Here's how the part is built. I have some questions about the finished solid (model axes, mm). Face numbers are marked on the shaded views. A direction names the side the tool comes from. Give positions to 0.01 mm unless a question says otherwise; leave off trailing zeros. Write each loop counter-clockwise with the first axis right and the second up, starting at its lowest first coordinate (ties: lowest second). Pieces come first, ordered by that corner, then holes. Notation, with made-up numbers: (80.5, -33.5) - (110.5, -33.5) arc R13 ccw to (110.5, -13.5) - close; hole circle Ø1 at (38.5, 16). An arc over 180 degrees is marked (long way). Use a Markdown table: item, result.
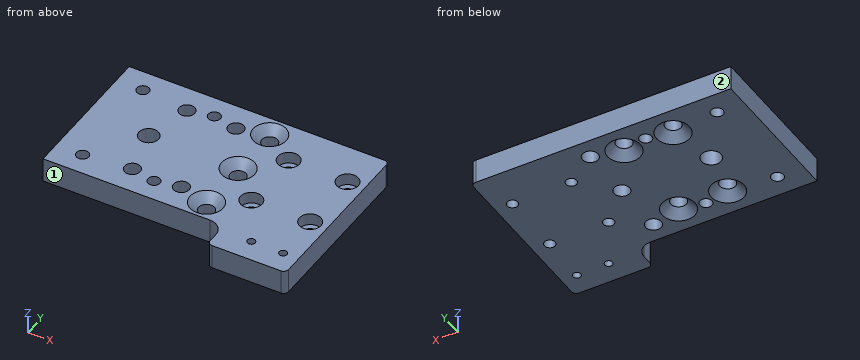
```python
from build123d import *

# Parameters (mm, degrees)
SCHIZZO1_W                                           = 52
SCHIZZO1_H                                           = 30
ESTRUSIONE_ESTRUSIONE1_DEPTH                         = 5
FORO_LAMATO_PER_VITE_M2_A_TESTA_CILINDRI_D           = 2.2
FORO_LAMATO_PER_VITE_M2_A_TESTA_CILINDRI_DEPTH       = 8.5
FORO_LAMATO_PER_VITE_M2_A_TESTA_CILINDRI_CBORE_D     = 4.4
FORO_LAMATO_PER_VITE_M2_A_TESTA_CILINDRI_CBORE_DEPTH = 2.4
FORO_LAMATO_PER_VITE_M2_A_TESTA_CILINDRI_TIP         = 0.660946681
FORO_SVASATO_PER_VITE_M3_1_D                         = 3.2
FORO_SVASATO_PER_VITE_M3_1_DEPTH                     = 8.5
FORO_SVASATO_PER_VITE_M3_1_CSINK_D                   = 6.72
FORO_SVASATO_PER_VITE_M3_1_CSINK_ANGLE               = 90
FORO_SVASATO_PER_VITE_M3_1_TIP                       = 0.96137699
FORO_4_0_4_1_D                                       = 4
FORO_4_0_4_1_DEPTH                                   = 8.5
FORO_4_0_4_1_TIP                                     = 1.201721238
FORO_FILETTATO_M3_1_D                                = 2.5
FORO_FILETTATO_M3_1_DEPTH                            = 8.5
FORO_FILETTATO_M3_1_TIP                              = 0.751075774
FORO_SVASATO_PER_VITE_M3_2_D                         = 3.2
FORO_SVASATO_PER_VITE_M3_2_CSINK_D                   = 6.72
FORO_SVASATO_PER_VITE_M3_2_CSINK_ANGLE               = 90
SCHIZZO11_W                                          = 15
SCHIZZO11_H                                          = 5
ESTRUSIONE_ESTRUSIONE2_DEPTH                         = 6
FORO_FILETTATO_M2_1_D                                = 1.6
FORO_FILETTATO_M2_1_DEPTH                            = 6
FORO_FILETTATO_M2_1_TIP                              = 0.480688495
SCHIZZO14_W                                          = 1
SCHIZZO14_H                                          = 5
ESTRUSIONE_ESTRUSIONE3_DEPTH                         = 36
RACCORDO1_R                                          = 1
RACCORDO2_R                                          = 3


with BuildPart() as part:
    # Schizzo1 → Estrusione-Estrusione1 (new body)
    with BuildSketch(Plane.XY):
        Rectangle(SCHIZZO1_W, SCHIZZO1_H)
    extrude(amount=ESTRUSIONE_ESTRUSIONE1_DEPTH)

    # Foro lamato per Vite M2 a testa cilindrica-1
    with Locations(Plane(origin=(11.5, 6.5, 5), x_dir=(1, 0, 0), z_dir=(0, 0, 1))):
        with Locations((0, 0), (12, 0), (0, -13), (12, -13)):
            CounterBoreHole(FORO_LAMATO_PER_VITE_M2_A_TESTA_CILINDRI_D / 2, FORO_LAMATO_PER_VITE_M2_A_TESTA_CILINDRI_CBORE_D / 2, FORO_LAMATO_PER_VITE_M2_A_TESTA_CILINDRI_CBORE_DEPTH, depth=FORO_LAMATO_PER_VITE_M2_A_TESTA_CILINDRI_DEPTH)
            with Locations((0, 0, -(FORO_LAMATO_PER_VITE_M2_A_TESTA_CILINDRI_DEPTH + FORO_LAMATO_PER_VITE_M2_A_TESTA_CILINDRI_TIP / 2))):  # 118° drill point
                Cone(0, FORO_LAMATO_PER_VITE_M2_A_TESTA_CILINDRI_D / 2, FORO_LAMATO_PER_VITE_M2_A_TESTA_CILINDRI_TIP, mode=Mode.SUBTRACT)

    # Foro svasato per Vite M3-1
    with Locations(Plane(origin=(0, 0, 0), x_dir=(-1, 0, 0), z_dir=(0, 0, -1))):
        with Locations((11, -9.5), (1, -9.5), (11, 9.5), (1, 9.5)):
            CounterSinkHole(FORO_SVASATO_PER_VITE_M3_1_D / 2, FORO_SVASATO_PER_VITE_M3_1_CSINK_D / 2, depth=FORO_SVASATO_PER_VITE_M3_1_DEPTH, counter_sink_angle=FORO_SVASATO_PER_VITE_M3_1_CSINK_ANGLE)
            with Locations((0, 0, -(FORO_SVASATO_PER_VITE_M3_1_DEPTH + FORO_SVASATO_PER_VITE_M3_1_TIP / 2))):  # 118° drill point
                Cone(0, FORO_SVASATO_PER_VITE_M3_1_D / 2, FORO_SVASATO_PER_VITE_M3_1_TIP, mode=Mode.SUBTRACT)

    # Foro Ø4.0 (4)-1
    with Locations(Plane(origin=(-13.23, 0, 5), x_dir=(1, 0, 0), z_dir=(0, 0, 1))):
        with Locations((0, 0)):
            Hole(FORO_4_0_4_1_D / 2, depth=FORO_4_0_4_1_DEPTH)
            with Locations((0, 0, -(FORO_4_0_4_1_DEPTH + FORO_4_0_4_1_TIP / 2))):  # 118° drill point
                Cone(0, FORO_4_0_4_1_D / 2, FORO_4_0_4_1_TIP, mode=Mode.SUBTRACT)

    # Foro filettato M3-1
    with Locations(Plane(origin=(-20.56, 10.5, 5), x_dir=(1, 0, 0), z_dir=(0, 0, 1))):
        with Locations((0, 0), (14.56, 0), (14.56, -21), (0, -21)):
            Hole(FORO_FILETTATO_M3_1_D / 2, depth=FORO_FILETTATO_M3_1_DEPTH)
            with Locations((0, 0, -(FORO_FILETTATO_M3_1_DEPTH + FORO_FILETTATO_M3_1_TIP / 2))):  # 118° drill point
                Cone(0, FORO_FILETTATO_M3_1_D / 2, FORO_FILETTATO_M3_1_TIP, mode=Mode.SUBTRACT)

    # Foro svasato per Vite M3-2 (through all)
    with Locations(Plane(origin=(5, 11, 5), x_dir=(1, 0, 0), z_dir=(0, 0, 1))):
        with Locations((0, 0), (0, -11), (0, -22)):
            CounterSinkHole(FORO_SVASATO_PER_VITE_M3_2_D / 2, FORO_SVASATO_PER_VITE_M3_2_CSINK_D / 2, counter_sink_angle=FORO_SVASATO_PER_VITE_M3_2_CSINK_ANGLE)

    # Schizzo11 → Estrusione-Estrusione2 (add)
    with BuildSketch(Plane.XZ.offset(15)):
        with Locations((18.5, 2.5)):
            Rectangle(SCHIZZO11_W, SCHIZZO11_H)
    extrude(amount=ESTRUSIONE_ESTRUSIONE2_DEPTH)

    # Foro filettato M2-1
    with Locations(Plane(origin=(17.35, -16.5, 5), x_dir=(1, 0, 0), z_dir=(0, 0, 1))):
        with Locations((0, 0), (6.5, 0)):
            Hole(FORO_FILETTATO_M2_1_D / 2, depth=FORO_FILETTATO_M2_1_DEPTH)
            with Locations((0, 0, -(FORO_FILETTATO_M2_1_DEPTH + FORO_FILETTATO_M2_1_TIP / 2))):  # 118° drill point
                Cone(0, FORO_FILETTATO_M2_1_D / 2, FORO_FILETTATO_M2_1_TIP, mode=Mode.SUBTRACT)

    # Schizzo14 → Estrusione-Estrusione3 (add)
    with BuildSketch(Plane.XZ.offset(21)):
        with Locations((26.5, 2.5)):
            Rectangle(SCHIZZO14_W, SCHIZZO14_H)
    extrude(amount=-ESTRUSIONE_ESTRUSIONE3_DEPTH)

    # Raccordo1
    raccordo1_edges = [part.edges().sort_by_distance(p)[0] for p in [
        (11, -21, 2.5),
        (27, -21, 2.5),
        (27, 15, 2.5),
    ]]
    fillet(raccordo1_edges, radius=RACCORDO1_R)

    # Raccordo2
    raccordo2_edges = [part.edges().sort_by_distance(p)[0] for p in [
        (11, -15, 2.5),
    ]]
    fillet(raccordo2_edges, radius=RACCORDO2_R)


solid = part.part
```
Item 1: For the marked faces 1 and 2, which set-ups out of +Z, -Z, +X, -X, +Y, -Y let a thin tool reach every point of the face, with its end or its side?
Values:
| item | result |
|---|---|
| face 1 | +Z, -Z, -X, -Y |
| face 2 | +Z, -Z, +X, -X, +Y |
Item 2: If we section it at C-C, the plane x = 4: Count the separate pieces of the cut face and the enclosed holes in it, plus the area to 3 significant figures.
Values:
| item | result |
|---|---|
| separate pieces | 4 |
| enclosed holes | 0 |
| area | 102 mm2 |
Item 3: Will these pins go through, and if not, where does the flat tip stop? pin 1 Ø2 at (x, y) = (-20.56, -10.5) entering from -Z; pin 2 Ø3 at (x, y) = (11.5, 6.5) entering from +Z.
Values:
| item | result |
|---|---|
| pin 1 | passes through |
| pin 2 | stops at z = 2.6 |
Item 4: I need wall thicknesses on line 1 along Y through (x, z) = (-20.56, 2.9); line 2 along Y through (x, z) = (17.35, 1.65); line 3 along Y through (x, z) = (-11, 3.15). Which ranges of each line are inside material? Lowest first, please. Write a range as [from, to].
Values:
| item | result |
|---|---|
| line 1 | y = [-15, -11.75], [-9.25, 9.25], [11.75, 15] |
| line 2 | y = [-21, -17.3], [-15.7, 15] |
| line 3 | y = [-15, -11.1], [-7.9, 7.9], [11.1, 15] |
Item 5: If we section it at A-A, the plane x = -20.56: Write out the boundary of the cut face in (y, z), plus the area to 3 significant figures.
Values:
| item | result |
|---|---|
| outline | (-15, 0) - (-11.75, 0) - (-11.75, 5) - (-15, 5) - close; (-9.25, 0) - (9.25, 0) - (9.25, 5) - (-9.25, 5) - close; (11.75, 0) - (15, 0) - (15, 5) - (11.75, 5) - close |
| area | 125 mm2 |
Item 6: If we section it at B-B, the plane y = 0: Write out the boundary of the cut face in (x, z).
Values:
| item | result |
|---|---|
| outline | (-26, 0) - (-15.23, 0) - (-15.23, 5) - (-26, 5) - close; (-11.23, 0) - (3.4, 0) - (3.4, 3.24) - (1.64, 5) - (-11.23, 5) - close; (6.6, 0) - (27, 0) - (27, 5) - (8.36, 5) - (6.6, 3.24) - close |
